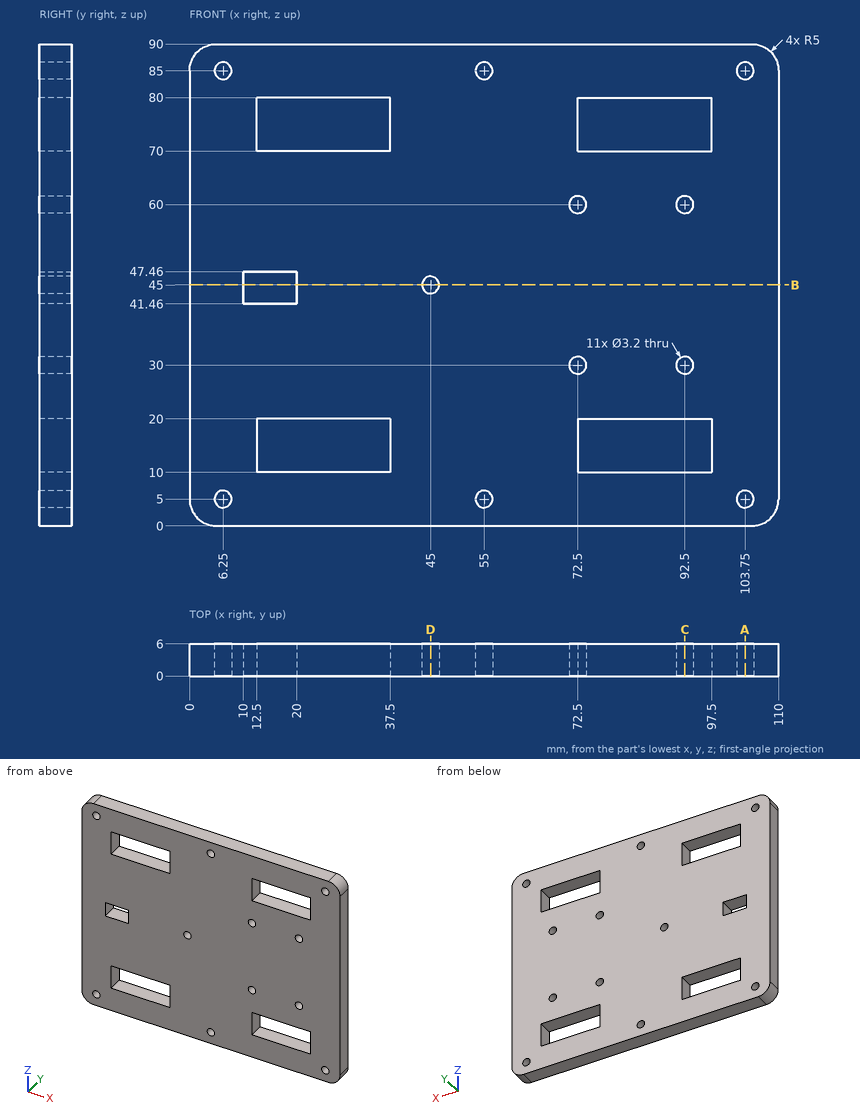
Job drawing, mm, ordinate dimensions from the low corner. One solid piece. Round coordinates to 2 decimals unless told otherwise and drop trailing zeros. Order: outer loops, then holes, each group sorted by start corner. A loop starts at its lowest first (then second) coordinate and runs counter-clockwise, first axis right, second up. Notation, with made-up numbers: (32.25, -14) - (68.25, -14) arc R13 cw to (68.25, 7) - close; hole circle Ø1 at (84.25, 37). An arc over 180 degrees is marked (long way). Use CSV: the item, a comma, the result in double quotes. Start each with the question number.
1) Saw through at B-B (z = 45). List the corners of the cut face in (x, y).
2) Wall check: L1, parallel to Z at x = 14.5, y = 4.95; L2, parallel to X at y = 4.2, z = 10.5; L3, parallel to Z at x = 6.25, y = 4.2. Give the ranges that are in metal, low to high. Write a range as [from, to].
3) Saw through at D-D (x = 45). List the corners of the cut face in (y, z).
4) Pin check, flat tip, straight feed: pin 1 Ø5 at (x, z) = (45, 45) entering from -Y. Stop position of the tip, or through.
5) Saw through at A-A (x = 103.75). List the corners of the cut face in (y, z), and give its area (3 significant figures).
6) Saw through at C-C (x = 92.5). List the corners of the cut face in (y, z).
Values follow:
1,outline,"(0, 0) - (10, 0) - (10, 6) - (0, 6) - close; (20, 0) - (43.4, 0) - (43.4, 6) - (20, 6) - close; (46.6, 0) - (110, 0) - (110, 6) - (46.6, 6) - close"
2,L1,"z = [0, 10], [20, 41.46], [47.46, 70], [80, 90]"
2,L2,"x = [0, 12.5], [37.5, 72.5], [97.5, 110]"
2,L3,"z = [0, 3.4], [6.6, 83.4], [86.6, 90]"
3,outline,"(0, 0) - (6, 0) - (6, 43.4) - (0, 43.4) - close; (0, 46.6) - (6, 46.6) - (6, 90) - (0, 90) - close"
4,pin 1,"stops at y = 0"
5,outline,"(0, 0) - (6, 0) - (6, 3.4) - (0, 3.4) - close; (0, 6.6) - (6, 6.6) - (6, 83.4) - (0, 83.4) - close; (0, 86.6) - (6, 86.6) - (6, 90) - (0, 90) - close"
5,area,"502 mm2"
6,outline,"(0, 0) - (6, 0) - (6, 10) - (0, 10) - close; (0, 20) - (6, 20) - (6, 28.4) - (0, 28.4) - close; (0, 31.6) - (6, 31.6) - (6, 58.4) - (0, 58.4) - close; (0, 61.6) - (6, 61.6) - (6, 70) - (0, 70) - close; (0, 80) - (6, 80) - (6, 90) - (0, 90) - close"
